```python
from build123d import *


with BuildPart() as f3:
    # F0 (on Top) → F3 section 0
    with BuildSketch(Plane.XY, mode=Mode.PRIVATE) as f3_s0:
        Polygon((-58.540445, 18.186722), (-57.854831, -17.46534), (-25.596111, 9.273707), (-16.032221, -15.40849), (23.73354, 0), (50.815396, -15.40849), (23.73354, 38.069602), (-10.20448, 9.273707), (-18.774686, 38.069602), align=None)
    loft([f3_s0.sketch, Vertex(-22.32356, 0, 100)])


solid = f3.part
```
Geometry: final body of the model. Coordinates: model frame, mm. A direction names the side the tool comes from. Give positions to 0.01 mm unless a question says otherwise; leave off trailing zeros. Loops run counter-clockwise (first coordinate to the right, second up) from the corner with the lowest first, then second, coordinate; pieces in that order, holes last. Notation, with made-up numbers: (37, -2) -> (78, -2) arc R20 cw to (78, 16) -> close; hole circle Ø8 at (79, 39). An arc over 180 degrees is marked (long way). Return JSON: item names as keys, results as strings.
Item 1: Section D-D, the plane y = 3.5. Output: boundary loops of the cut face in (x, z).
Filled in:
{"outline": "(-58.26, 0) -> (-32.56, 0) -> (-23.56, 62.26) -> (-23.36, 0) -> (41.24, 0) -> (-18.09, 90.81) -> (-17.75, 62.26) -> (-22, 90.81) -> (-29.29, 80.76) -> close"}
Item 2: Line query: line 1 (X direction, y = 17.5, z = 4.5); line 2 (X direction, y = 25, z = 10.5); line 3 (Y direction, x = 24, z = 14.5). Output: solid intervals per line, ascending.
Filled in:
{"line 1": "-56.65 to -13.32, -0.56 to 31.21", "line 2": "-37.29 to -16.45, 8.21 to 23.49", "line 3": "-3.95 to 18.84"}
Item 3: Mould query, pull axis Z, two halves, no side actions, for faces 1 (the flat face through (-34.24, 20, 28.48)), 2 (the flat face through (-3, 7, 0)), 3 (the flat face through (18.453, -5.306, 31.715)). Classes: released by +Z, released by -Z, zero draft, split by the parting line, or undercut.
Filled in:
{"face 1": "released by +Z", "face 2": "released by -Z", "face 3": "undercut"}
Item 4: Section B-B, the plane z = 57. Output: boundary loops of the cut face in (x, y), plus the area to 3 significant figures.
Filled in:
{"outline": "(-37.9, 7.82) -> (-37.6, -7.51) -> (-23.73, 3.99) -> (-19.62, -6.63) -> (-2.52, 0) -> (9.13, -6.63) -> (-2.52, 16.37) -> (-17.11, 3.99) -> (-20.8, 16.37) -> close", "area": "575 mm^2"}
Item 5: Access query for faces 4 (the flat face through (19.646, 9.399, 28.478)), 5 (the flat face through (-7.2, -6.9, 28.5)), 6 (the flat face through (-36.036, -4.125, 39.589)). Directions: +Z, -Z, +X, -X, +Y, -Y. A direction counts if a zero-diameter tool reaches every point of the face in a straight line with its end or side. Return the directions, or none.
Filled in:
{"face 4": "+Z, +X, +Y", "face 5": "-Y", "face 6": "-Z, -Y"}
Item 6: Pin query (flat end, axial travel): P1, Ø8, axis at y = -8.5, z = 83.5, coming from the -X side; P2, Ø4, axis at y = 30, z = 24, coming from the +X side; P3, Ø4, axis at x = 8, y = 5, coming from the +Z side; P4, Ø8, axis at x = 3.5, z = 56, coming from the +Y side. Return the tip coordinate at first contact, or that it passes through.
Filled in:
{"P1": "through", "P2": "x = 13.79", "P3": "z = 53.14", "P4": "y = 15.21"}
Item 7: Section A-A, the plane y = 13. Output: boundary loops of the cut face in (x, z).
Filled in:
{"outline": "(-58.44, 0) -> (-11.31, 0) -> (-21.11, 65.85) -> (-48.21, 28.52) -> close; (-6.6, 65.85) -> (-5.81, 0) -> (36.43, 0) -> close"}
Item 8: Section C-C, the plane x = -2. Output: boundary loops of the cut face in (y, z).
Filled in:
{"outline": "(-9.97, 0) -> (16.24, 0) -> (16.8, 55.87) -> (-4.28, 72.21) -> (0, 55.87) -> close"}
